from build123d import *

# Parameters (mm, degrees)
F0_W     = 145
F0_H     = 70
F0_W_2   = 135
F0_H_2   = 60
F1_DEPTH = 125
F2_DEPTH = 5
F3_R     = 15
F5_DEPTH = 5
F6_SIZE  = 10


with BuildPart() as f1:
    # F0 (on Top) → F1 (new body)
    with BuildSketch(Plane.XY):
        Rectangle(F0_W, F0_H)
        Rectangle(F0_W_2, F0_H_2, mode=Mode.SUBTRACT)
    extrude(amount=F1_DEPTH)

    # F0 (on Top) → F2 (join)
    with BuildSketch(Plane.XY):
        Rectangle(F0_W_2, F0_H_2)
    extrude(amount=F2_DEPTH)

    # F3
    f3_edges = [f1.edges().sort_by_distance(p)[0] for p in [
        (-72.5, 35, 62.5),
        (-67.5, 30, 65),
        (-67.5, -30, 65),
        (-72.5, -35, 62.5),
        (72.5, -35, 62.5),
        (67.5, -30, 65),
        (67.5, 30, 65),
        (72.5, 35, 62.5),
    ]]
    fillet(f3_edges, radius=F3_R)

    # F4 (on face) → F5 (join)
    with BuildSketch(Plane(origin=(0, 0, 0), x_dir=(1, 0, 0), z_dir=(0, 0, -1))):
        with BuildLine():
            Line((57.5, 55), (-57.5, 55))
            ThreePointArc((-57.5, 55), (-82.2487373415, 44.7487373415), (-92.5, 20))
            Line((-92.5, 20), (-92.5, -20))
            ThreePointArc((-92.5, -20), (-82.2487373415, -44.7487373415), (-57.5, -55))
            Line((-57.5, -55), (57.5, -55))
            ThreePointArc((57.5, -55), (82.2487373415, -44.7487373415), (92.5, -20))
            Line((92.5, -20), (92.5, 20))
            ThreePointArc((92.5, 20), (82.2487373415, 44.7487373415), (57.5, 55))
        make_face()
    extrude(amount=-F5_DEPTH)

    # F6
    f6_edges = [f1.edges().sort_by_distance(p)[0] for p in [
        (-68.106602, 30.606602, 5),
    ]]
    chamfer(f6_edges, length=F6_SIZE)


solid = f1.part
Model file for the job. Use its own axes, mm. A direction names the side the tool comes from. Give positions to 0.01 mm unless a question says otherwise; leave off trailing zeros. Order: outer loops, then holes, each group sorted by start corner. A loop starts at its lowest first (then second) coordinate and runs counter-clockwise, first axis right, second up. Notation, with made-up numbers: (9.5, 69) - (61.5, 69) arc R15 ccw to (61.5, 97) - close; hole circle Ø10 at (-24.5, 7). An arc over 180 degrees is marked (long way). Write item = value, one per line. Start each with the question number.
1. Drop flat-ended pins along their axis: P1, Ø10, axis at x = 43.5, z = 98.5, coming from the -Y side; P2, Ø15, axis at y = -6.5, z = 63.5, coming from the +X side; P3, Ø3, axis at x = 72, z = 106.5, coming from the -Y side. Give the stop position or say it passes through.
2. Two-plate mould, pull along Y, no slides. Class faces 4 (the cylindrical face through (82.519, -44.475, 2.465)), 5 (the flat face through (-67.5, 0, 64)), 6 (the flat face through (-1, -1, 0)): pulls with the +Y half, pulls with the -Y half, needs draft (parallel to the pull), parting line crosses it, or undercut.
3. Cut at C-C, the plane x = -11. List the corners of the cut face in (y, z).
4. Cut at A-A, the plane z = 34.5. List the corners of the cut face in (x, y).
5. Probe line 1 along Y through (x, z) = (-50, 53); line 2 along X through (y, z) = (1.5, 107); line 3 along Y through (x, z) = (6.5, 9). List the from-to ranges inside material, lowest first.
6. Cut at D-D, the plane z = 11.5. List the corners of the cut face in (x, y).
7. Cut at B-B, the plane y = 7. List the corners of the cut face in (x, z), and give its area (4 significant figures).
8. Which spindle directions (+Z, -Z, +X, -X, +Y, -Y) get a long thin tool onto all of the face, cutting with end or side? Do faces 1 (the cylindrical face through (-62.99, -25.72, 65.84)), 2 (the flat face through (-1, -35, 69)), 3 (the flat face through (72.5, 0, 69)). Say none if no direction does.
Taken from the geometry:
q1.P1 = -35
q1.P2 = 72.5
q1.P3 = -27.48
q2.face_4 = pulls with the -Y half
q2.face_5 = undercut
q2.face_6 = needs draft
q3.outline = (-55, 0) - (55, 0) - (55, 5) - (45, 5) - (35, 15) - (35, 125) - (30, 125) - (30, 5) - (-30, 5) - (-30, 125) - (-35, 125) - (-35, 15) - (-45, 5) - (-55, 5) - close
q4.outline = (-72.5, -20) arc R15 ccw to (-57.5, -35) - (57.5, -35) arc R15 ccw to (72.5, -20) - (72.5, 20) arc R15 ccw to (57.5, 35) - (-57.5, 35) arc R15 ccw to (-72.5, 20) - close; hole (-67.5, -15) arc R15 ccw to (-52.5, -30) - (52.5, -30) arc R15 ccw to (67.5, -15) - (67.5, 15) arc R15 ccw to (52.5, 30) - (-52.5, 30) arc R15 ccw to (-67.5, 15) - close
q5.line_1 = -35 to -30, 30 to 35
q5.line_2 = -72.5 to -67.5, 67.5 to 72.5
q5.line_3 = -41 to -30, 30 to 41
q6.outline = (-76, -20) arc R18.5 ccw to (-57.5, -38.5) - (57.5, -38.5) arc R18.5 ccw to (76, -20) - (76, 20) arc R18.5 ccw to (57.5, 38.5) - (-57.5, 38.5) arc R18.5 ccw to (-76, 20) - close; hole (-67.5, -15) arc R15 ccw to (-52.5, -30) - (52.5, -30) arc R15 ccw to (67.5, -15) - (67.5, 15) arc R15 ccw to (52.5, 30) - (-52.5, 30) arc R15 ccw to (-67.5, 15) - close
q7.outline = (-92.5, 0) - (92.5, 0) - (92.5, 5) - (82.5, 5) - (72.5, 15) - (72.5, 125) - (67.5, 125) - (67.5, 5) - (-67.5, 5) - (-67.5, 125) - (-72.5, 125) - (-72.5, 15) - (-82.5, 5) - (-92.5, 5) - close
q7.area = 2,225 mm²
q8.face_1 = +Z
q8.face_2 = +Z, +X, -X, -Y
q8.face_3 = +Z, +X, +Y, -Y
